The drawing under review shows one solid part. Ordinate dimensions are in mm from its lowest x, y, z. A direction names the side the tool comes from. Give positions to 0.01 mm unless a question says otherwise; leave off trailing zeros. Write each loop counter-clockwise with the first axis right and the second up, starting at its lowest first coordinate (ties: lowest second). Pieces come first, ordered by that corner, then holes.
Q1. For line 1 (Y direction, x = 32.7, z = 15); line 2 (X direction, y = 23.5, z = 13.95); line 3 (Y direction, x = 33.5, z = 14), list the stretches that pass through material, from the lowest coordinate up.
Q2. We need section A-A (y = 23.5). Write out the cut boundary in (x, z).
Q3. Insertion check: P1, Ø5, axis at x = 12.7, y = 3.5, coming from the -Z side; P2, Ø1, axis at x = 38, y = 24.5, coming from the +Z side; P3, Ø8, axis at x = 40.5, z = 2.5, coming from the -Y side; P4, Ø1.9, axis at x = 12.7, y = 23.5, coming from the +Z side (3 decimals). Each pin has a flat end and moves straight along its axis. Give the tip position at first contact, or say it passes through.
Q4. We need section B-B (x = 12.7). Give the number of separate pieces and of enclosed holes in the cut face, then the cut area to 3 significant figures.
Q5. We need section C-C (x = 6). Write out the cut boundary in (y, z), then the cut area to 3 significant figures.
Q6. Machinability: for the marked faces 4 and 5, which of the approach directions +Z, -Z, +X, -X, +Y, -Y give a long, thin tool a straight path to every point of the face, cutting with its end or side? Answer none if there is none.
Q7. We need section D-D (z = 10). Write out the cut boundary in (x, y), then the cut area to 3 significant figures.
Q8. Mouldability with a two-part tool opening along X and no side actions: class the marked faces 1, 2 and 3 as released by +X, released by -X, zero draft, split by the parting line, or undercut.
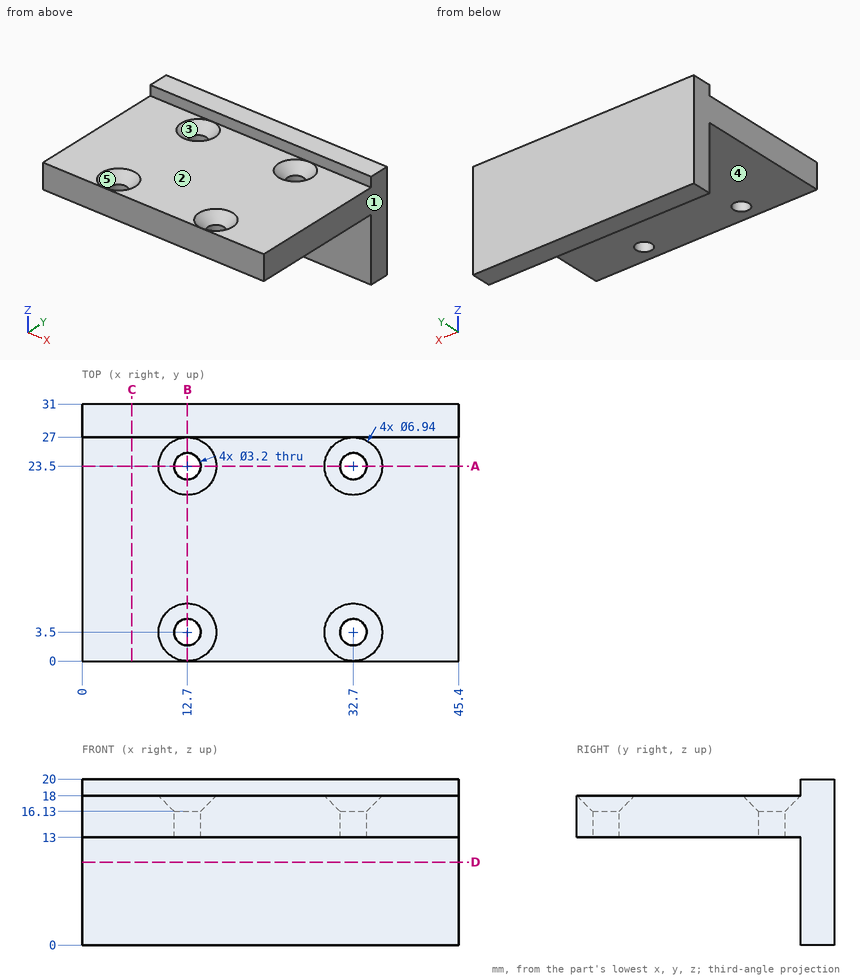
Computed:
1. line 1: y = 0 to 1.9, 5.1 to 21.9, 25.1 to 31
1. line 2: x = 0 to 11.1, 14.3 to 31.1, 34.3 to 45.4
1. line 3: y = 0 to 2.11, 4.89 to 22.11, 24.89 to 31
2. outline: (0, 13) - (11.1, 13) - (11.1, 16.13) - (9.23, 18) - (0, 18) - close; (14.3, 13) - (31.1, 13) - (31.1, 16.13) - (29.23, 18) - (16.17, 18) - (14.3, 16.13) - close; (34.3, 13) - (45.4, 13) - (45.4, 18) - (36.17, 18) - (34.3, 16.13) - close
3. P1: stops at z = 13
3. P2: stops at z = 18
3. P3: stops at y = 27
3. P4: passes through
4. separate pieces: 3
4. enclosed holes: 0
4. area: 176 mm2
5. outline: (0, 13) - (27, 13) - (27, 0) - (31, 0) - (31, 20) - (27, 20) - (27, 18) - (0, 18) - close
5. area: 215 mm2
6. face 4: -Z, +X, -X, -Y
6. face 5: +Z
7. outline: (0, 27) - (45.4, 27) - (45.4, 31) - (0, 31) - close
7. area: 182 mm2
8. face 1: released by +X
8. face 2: zero draft
8. face 3: undercut
